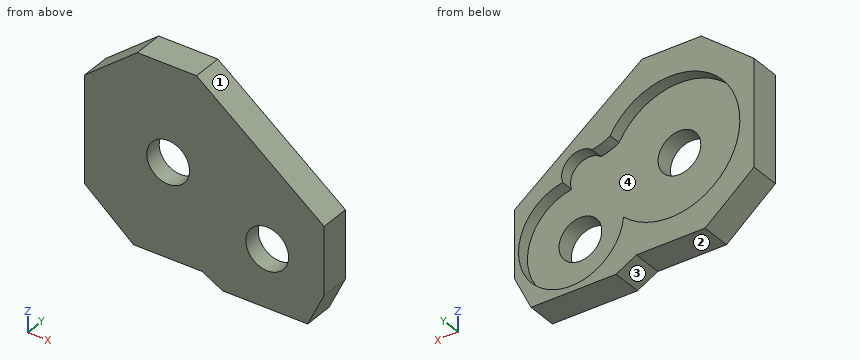
```python
from build123d import *

# Parameters (mm, degrees)
EXTRUDE_START       = -2
EXTRUDE_1_DEPTH     = 12
CUT_EXTRUDE_1_DEPTH = 5
SKETCH_4_R          = 8.5
CUT_EXTRUDE_2_DEPTH = 109.143461437


with BuildPart() as part:
    # Эскиз1 → Вытянуть1 (new body)
    with BuildSketch(Plane(origin=(0, 0, 0), x_dir=(1, 0, 0), z_dir=(0, 1, 0)).offset(EXTRUDE_START)):
        Polygon((41.234335961, 16.139303033), (49.33132622, 20.576367476), (83.159652077, 20.576367476), (89.695898477, 7.004834382), (89.695898477, -19.904859962), (38.978411799, -59.208563976), (15.42620007, -59.208563976), (-5.538491663, -42.514725177), (-5.538491663, -0.189156064), (13.914350861, 16.139303033), align=None)
    extrude(amount=EXTRUDE_1_DEPTH)

    # Эскиз2 → Вырез-Вытянуть1 (cut)
    with BuildSketch(Plane(origin=(0, 10, 0), x_dir=(1, 0, 0), z_dir=(0, 1, 0))):
        with BuildLine():
            ThreePointArc((46.353434454, -0.558740061), (0.463282904, -25.097768311), (51.691914237, -34.246388345))
            ThreePointArc((51.691914237, -34.246388345), (55.121981017, -32.508830766), (58.84329247, -31.541201954))
            ThreePointArc((58.84329247, -31.541201954), (67.819533531, -31.785998768), (70.560678986, -23.235036795))
            ThreePointArc((70.560678986, -23.235036795), (81.500890347, 12.702706564), (46.353434454, -0.558740061))
        make_face()
    extrude(amount=-CUT_EXTRUDE_1_DEPTH, mode=Mode.SUBTRACT)

    # Эскиз4 → Вырез-Вытянуть2 (cut, through all)
    with BuildSketch(Plane.XZ.offset(2)):
        with Locations(Location((27.688571463, 21.162784436, 0), (0, 0, 270))):
            Circle(SKETCH_4_R)
        with Locations(Location((67.068947784, 2.498184147, 0), (0, 0, 270))):
            Circle(SKETCH_4_R)
    extrude(amount=-CUT_EXTRUDE_2_DEPTH, mode=Mode.SUBTRACT)


solid = part.part
```
Read the model definition and answer for the solid it produces. Units are mm, in the model's axes. Face numbers are marked on the shaded views. Coordinates: 2 decimals unless noted, no trailing zeros. Loops run counter-clockwise (first coordinate to the right, second up) from the corner with the lowest first, then second, coordinate; pieces in that order, holes last.
(1) Consider line 1 along X through (y, z) = (2, 2.5); line 2 along Y through (x, z) = (35.5, 30); line 3 along Z through (x, y) = (54, 9). Determine where each line is inside the solid, lowest interval first.
Solution:
line 1: x = -5.54 to 58.57, 75.57 to 89.7
line 2: y = -2 to 5
line 3: z = -20.58 to -13.68, 32.98 to 47.57
(2) Flat-ended cylindrical pins translate along their axes: pin 1 Ø1.5 at (x, y) = (6.5, 5.5) entering from +Z; pin 2 Ø1 at (x, y) = (24, 3.5) entering from -Z; pin 3 Ø5 at (y, z) = (3, 49) entering from +X. Find the tip coordinate at first contact, or state that the pin passes through.
Solution:
pin 1: stops at z = 52.7
pin 2: stops at z = -16.14
pin 3: stops at x = 55.38
(3) The part is cut by section A-A (z = 3). Determine the outline of the cut face in (x, y).
Solution:
outline: (-5.54, -2) - (58.58, -2) - (58.58, 5) - (6.64, 5) - (6.64, 10) - (-5.54, 10) - close; (75.55, -2) - (89.7, -2) - (89.7, 10) - (88.12, 10) - (88.12, 5) - (75.55, 5) - close
(4) The part is cut by section C-C (y = 0.5). Determine the outline of the cut face in (x, z), and give its area (3 significant figures).
Solution:
outline: (-5.54, 0.19) - (13.91, -16.14) - (41.23, -16.14) - (49.33, -20.58) - (83.16, -20.58) - (89.7, -7) - (89.7, 19.9) - (38.98, 59.21) - (15.43, 59.21) - (-5.54, 42.51) - close; hole circle Ø17 at (27.69, 21.16); hole circle Ø17 at (67.07, 2.5)
area: 5,540 mm2
(5) The part is cut by section D-D (x = 79). Determine the outline of the cut face in (y, z).
Solution:
outline: (-2, -20.58) - (10, -20.58) - (10, -14.71) - (5, -14.71) - (5, 19.86) - (10, 19.86) - (10, 28.19) - (-2, 28.19) - close
(6) The part is cut by section B-B (x = 20.5). Determine the outline of the cut face in (y, z).
Solution:
outline: (-2, -16.14) - (10, -16.14) - (10, -5.81) - (5, -5.81) - (5, 16.63) - (-2, 16.63) - close; (-2, 25.7) - (5, 25.7) - (5, 47.38) - (10, 47.38) - (10, 59.21) - (-2, 59.21) - close
(7) The mould has two halves that part along X. Classify the marked faces 1, 2, 3 and 4: released by +X, released by -X, zero draft, split by the parting line, or undercut.
Solution:
face 1: released by +X
face 2: zero draft
face 3: released by -X
face 4: undercut
